Geometry: see drawing. Coordinates: mm, zero at the bounding-box minimum. Give positions to 0.01 mm unless a question says otherwise; leave off trailing zeros. Write each loop counter-clockwise with the first axis right and the second up, starting at its lowest first coordinate (ties: lowest second). Pieces come first, ordered by that corner, then holes. Notation, with made-up numbers: (75, 63) - (82, 63) arc R6 ccw to (82, 74) - close; hole circle Ø10 at (-32.75, -24). An arc over 180 degrees is marked (long way). One line per question, with ' | ' between items. Start each with the question number.
(1) Section C-C, the plane y = 4.25. Return loops of the section in (x, z).
(2) Ray query, line 1 (X direction, y = 3, z = 35.5); line 2 (Y direction, x = 7.5, z = 42); line 3 (Z direction, x = 5.5, y = 1.25). Return the intervals inside material, ascending. Write a range as [from, to].
(3) Section D-D, the plane z = 165. Return loops of the section in (x, y), plus the area to 3 significant figures.
(4) Pin query (flat end, axial travel): pin 1 (10 mm diameter, centred on x = 7.5, z = 88, fed in from +Y); pin 2 (5 mm diameter, centred on x = 16, z = 123, fed in from +Y); pin 3 (2 mm diameter, centred on y = 1, z = 117.5, fed in from -X); pin 4 (1.4 mm diameter, centred on y = 0.5, z = 119.5, fed in from +X). Return the tip coordinate at first contact, or that it passes through.
(5) Section A-A, the plane z = 23.5. Return loops of the section in (x, y), plus the area to 3 significant figures.
(6) Section B-B, the plane x = 18. Return loops of the section in (y, z), plus the area to 3 significant figures.
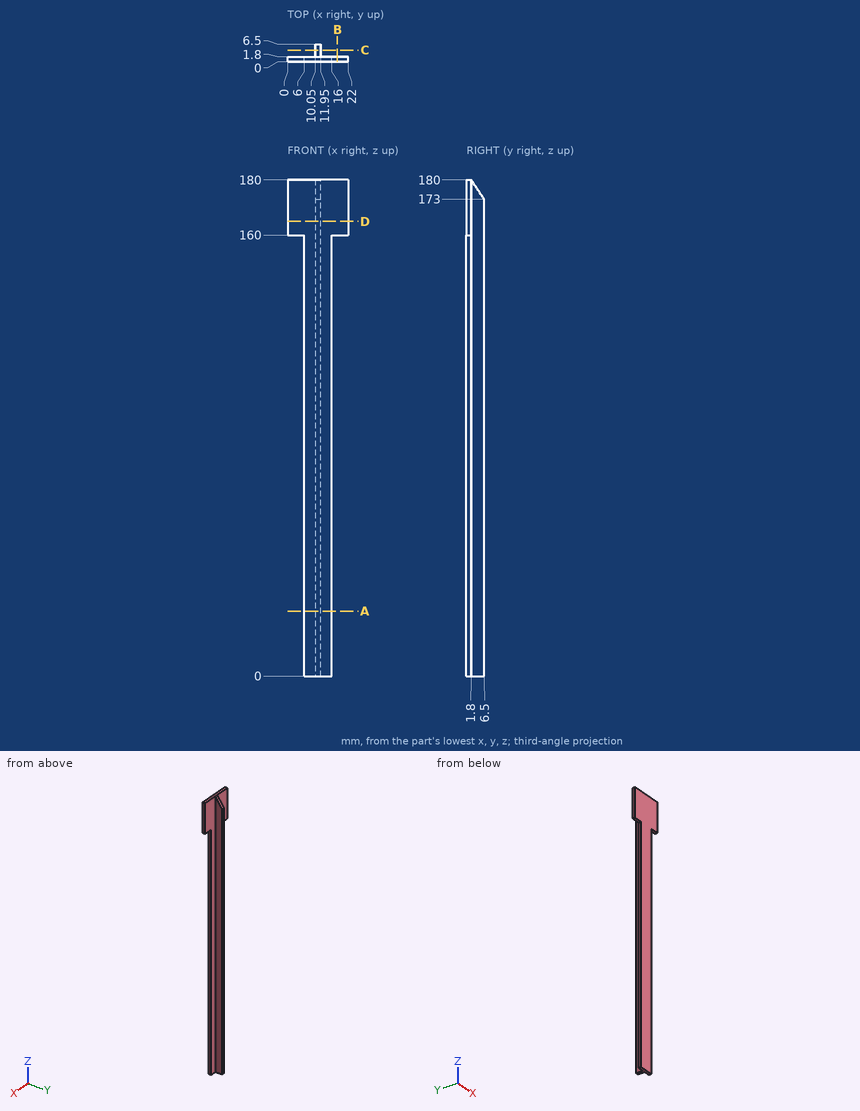
Check sheet entries:
1) outline: (10.05, 0) - (11.95, 0) - (11.95, 176.35) - (10.05, 176.35) - close
2) line 1: [10.05, 11.95] | line 2: [0, 1.8] | line 3: [160, 180]
3) outline: (0, 0) - (22, 0) - (22, 1.8) - (11.95, 1.8) - (11.95, 6.5) - (10.05, 6.5) - (10.05, 1.8) - (0, 1.8) - close | area: 48.5 mm²
4) pin 1: y = 6.5 | pin 2: y = 1.8 | pin 3: x = 6 | pin 4: x = 16
5) outline: (6, 0) - (16, 0) - (16, 1.8) - (11.95, 1.8) - (11.95, 6.5) - (10.05, 6.5) - (10.05, 1.8) - (6, 1.8) - close | area: 26.9 mm²
6) outline: (0, 160) - (1.8, 160) - (1.8, 180) - (0, 180) - close | area: 36.0 mm²
